from build123d import *

# Parameters (mm, degrees)
F0_W      = 127
F0_H      = 152.4
F1_DEPTH  = 76.2
F2_T      = -1.4986
F3_W      = 1.4986
F3_H      = 149.4028
F5_DEPTH  = 74.7014
F6_DEPTH  = 19.05
F8_DEPTH  = 19.05
F9_W      = 103.4542
F9_H      = 1.4986
F10_DEPTH = 74.7014


# Not quite as in the source:
# - an extrude ends at something that could not be found from the text; its depth is read off the source's solid


with BuildPart() as f1:
    # F0 (on Top) → F1 (new body)
    with BuildSketch(Plane.XY):
        Rectangle(F0_W, F0_H)
    extrude(amount=F1_DEPTH)

    # F2
    f2_openings = [f1.faces().sort_by_distance(p)[0] for p in [
        (0, 0, 76.2),
    ]]
    offset(amount=F2_T, openings=f2_openings)

    # F3 (on face) → F5 (join, through all)
    with BuildSketch(Plane.XY.offset(1.4986)):
        with Locations((-42.2021, 0)):
            Rectangle(F3_W, F3_H)
    extrude(amount=F5_DEPTH)

    # F4 (on face) → F6 (join, through all)
    with BuildSketch(Plane.YZ.offset(-62.0014)):
        Polygon((-74.7014, 74.7014), (74.7014, 36.6014), (74.7014, 38.1), (-74.7014, 76.2), align=None)
    extrude(amount=F6_DEPTH)

    # F7 (on face) → F8 (join, through all)
    with BuildSketch(Plane(origin=(-42.9514, 0, 0), x_dir=(0, -1, 0), z_dir=(-1, 0, 0))):
        Polygon((-74.7014, 76.2), (-74.7014, 38.1), (-62.0014, 41.3386943217), (-62.0014, 76.2), align=None)
    extrude(amount=F8_DEPTH)

    # F9 (on face) → F10 (join, through all)
    with BuildSketch(Plane.XY.offset(1.4986)):
        with Locations((10.2743, 0)):
            Rectangle(F9_W, F9_H)
    extrude(amount=F10_DEPTH)


solid = f1.part
Geometry: final body of the model. Coordinates: model frame, mm. A direction names the side the tool comes from. Give positions to 0.01 mm unless a question says otherwise; leave off trailing zeros. Order: outer loops, then holes, each group sorted by start corner. A loop starts at its lowest first (then second) coordinate and runs counter-clockwise, first axis right, second up. Notation, with made-up numbers: (86, 41.5) -> (141, 41.5) arc R11 ccw to (141, 62.5) -> close; hole circle Ø5 at (20, 18). An arc over 180 degrees is marked (long way). Put each result on its own line as item: value.
Q1. Material intervals for L1, parallel to X at y = 13, z = 26; L2, parallel to Y at x = 15.5, z = 57.5; L3, parallel to Z at x = -30, y = -64, sorted ascending.
Here are the results:
L1: x = -63.5 to -62, -42.95 to -41.45, 62 to 63.5
L2: y = -76.2 to -74.7, -0.75 to 0.75, 74.7 to 76.2
L3: z = 0 to 1.5
Q2. Section C-C, the plane z = 53. Return loops of the section in (x, y), then the cut area to 3 significant figures.
Here are the results:
outline: (-63.5, -76.2) -> (63.5, -76.2) -> (63.5, 76.2) -> (-63.5, 76.2) -> close; hole (-62, -74.7) -> (-42.95, -74.7) -> (-42.95, 10.4) -> (-62, 10.4) -> close; hole (-62, 16.27) -> (-42.95, 16.27) -> (-42.95, 62) -> (-62, 62) -> close; hole (-41.45, -74.7) -> (62, -74.7) -> (62, -0.75) -> (-41.45, -0.75) -> close; hole (-41.45, 0.75) -> (62, 0.75) -> (62, 74.7) -> (-41.45, 74.7) -> close
area: 1,560 mm^2
Q3. Reachability of faces 4 (the face through (-1, 1, 0)), 5 (the face through (-62.001, 23, 66)), 6 (the face through (-62.001, -1, 29)) from +Z, -Z, +X, -X, +Y, -Y: full face, straight path, thin tool, end or side. Return the list, or none.
Here are the results:
face 4: -Z, +X, -X, +Y, -Y
face 5: +Z
face 6: none
Q4. Section A-A, the plane x = 40.5. Return loops of the section in (y, z), then the cut area to 3 significant figures.
Here are the results:
outline: (-76.2, 0) -> (76.2, 0) -> (76.2, 76.2) -> (74.7, 76.2) -> (74.7, 1.5) -> (0.75, 1.5) -> (0.75, 76.2) -> (-0.75, 76.2) -> (-0.75, 1.5) -> (-74.7, 1.5) -> (-74.7, 76.2) -> (-76.2, 76.2) -> close
area: 564 mm^2
Q5. Section D-D, the plane y = 36. Return loops of the section in (x, z).
Here are the results:
outline: (-63.5, 0) -> (63.5, 0) -> (63.5, 76.2) -> (62, 76.2) -> (62, 1.5) -> (-41.45, 1.5) -> (-41.45, 76.2) -> (-42.95, 76.2) -> (-42.95, 47.97) -> (-62, 47.97) -> (-62, 76.2) -> (-63.5, 76.2) -> close; hole (-62, 1.5) -> (-42.95, 1.5) -> (-42.95, 46.47) -> (-62, 46.47) -> close
Q6. Draft query along Y for faces 1 (the face through (-23, 0, 76.2)), 2 (the face through (62.001, -38, 38)), 3 (the face through (-1, -76.2, 38)). Return one class per face: released by +Y, released by -Y, zero draft, split by the parting line, or undercut.
Here are the results:
face 1: zero draft
face 2: undercut
face 3: released by -Y
Q7. Pin query (flat end, axial travel): pin 1 (2 mm diameter, centred on x = 16, y = -50.5, fed in from -Z); pin 2 (10 mm diameter, centred on x = -5, y = 56.5, fed in from +Z). Return the tip coordinate at first contact, or that it passes through.
Here are the results:
pin 1: stops at z = 0
pin 2: stops at z = 1.5
Q8. Section B-B, the plane x = -56. Return loops of the section in (y, z).
Here are the results:
outline: (-76.2, 0) -> (76.2, 0) -> (76.2, 76.2) -> (62, 76.2) -> (62, 41.34) -> (-74.7, 76.2) -> (-76.2, 76.2) -> close; hole (-74.7, 1.5) -> (74.7, 1.5) -> (74.7, 36.6) -> (-74.7, 74.7) -> close
